Geometry: see drawing. Coordinates: mm, zero at the bounding-box minimum. A direction names the side the tool comes from. Round coordinates to 2 decimals unless told otherwise and drop trailing zeros. Loops run counter-clockwise (first coordinate to the right, second up) from the corner with the lowest first, then second, coordinate; pieces in that order, holes last.
(1) First-contact query: pin 1 Ø1.5 at (x, y) = (20, 20.5) entering from -Z; pin 2 Ø1.5 at (y, z) = (19.5, 11) entering from +X; pin 3 Ø8 at (x, y) = (25, 4.5) entering from +Z (3 decimals). Flat tips, straight axial feed; report the tip coordinate or a pass-through.
(2) Access query for the marked faces 1 and 2. Directions: +Z, -Z, +X, -X, +Y, -Y. A direction counts if a zero-diameter tool reaches every point of the face in a straight line with its end or side. Return the directions, or none.
(3) Draft query along Z for the marked faces 3, 4 and 5. Return one class per face: released by +Z, released by -Z, zero draft, split by the parting line, or undercut.
(4) Line query: line 1 (X direction, y = 4.5, z = 18); line 2 (Y direction, x = 12.5, z = 10.5); line 3 (X direction, y = 16, z = 20). Output: solid intervals per line, ascending.
(5) Cut plane D-D, the plane x = 20. Output: boundary loops of the cut face in (y, z).
(6) Cut plane C-C, the plane z = 20. Output: boundary loops of the cut face in (x, y).
(7) Cut plane A-A, the plane z = 4. Output: boundary loops of the cut face in (x, y).
(8) Cut plane B-B, the plane x = 4. Output: boundary loops of the cut face in (y, z), and give its area (3 significant figures).
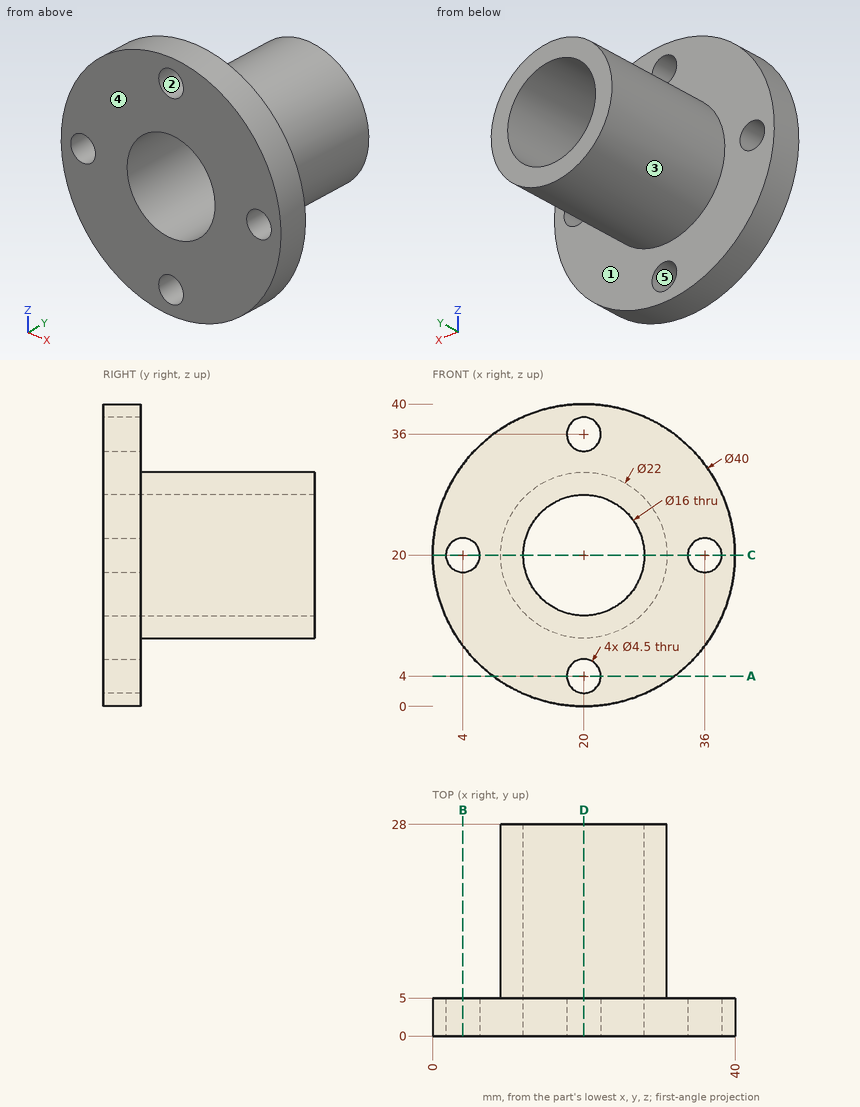
Reported:
1. pin 1: stops at z = 9
1. pin 2: stops at x = 27.28
1. pin 3: stops at z = 39.975
2. face 1: +Y
2. face 2: +Y, -Y
3. face 3: split by the parting line
3. face 4: zero draft
3. face 5: undercut
4. line 1: x = 0.1 to 2.97, 5.03 to 12.25, 27.75 to 34.97, 37.03 to 39.9
4. line 2: y = 0 to 5
4. line 3: x = 9 to 12, 28 to 31
5. outline: (0, 0) - (5, 0) - (5, 1.75) - (0, 1.75) - close; (0, 6.25) - (5, 6.25) - (5, 9) - (28, 9) - (28, 12) - (0, 12) - close; (0, 28) - (28, 28) - (28, 31) - (5, 31) - (5, 33.75) - (0, 33.75) - close; (0, 38.25) - (5, 38.25) - (5, 40) - (0, 40) - close
6. outline: (0, 0) - (1.75, 0) - (1.75, 5) - (0, 5) - close; (6.25, 0) - (12, 0) - (12, 28) - (9, 28) - (9, 5) - (6.25, 5) - close; (28, 0) - (33.75, 0) - (33.75, 5) - (31, 5) - (31, 28) - (28, 28) - close; (38.25, 0) - (40, 0) - (40, 5) - (38.25, 5) - close
7. outline: (8, 0) - (17.75, 0) - (17.75, 5) - (8, 5) - close; (22.25, 0) - (32, 0) - (32, 5) - (22.25, 5) - close
8. outline: (0, 8) - (5, 8) - (5, 17.75) - (0, 17.75) - close; (0, 22.25) - (5, 22.25) - (5, 32) - (0, 32) - close
8. area: 97.5 mm2
